from build123d import *

# Parameters (mm, degrees)
MODEL_R             = 1.25
BOSS_EXTRUDE1_DEPTH = 30
SKETCH1_R           = 2
BOSS_EXTRUDE3_DEPTH = 33
SKETCH3_W           = 38.889950408
SKETCH3_H           = 20
BOSS_EXTRUDE6_DEPTH = 3


with BuildPart() as part:
    # Model → Boss-Extrude1 (new body)
    with BuildSketch(Plane.XY):
        Polygon((29.652943866, 16.209286981), (29.652943866, 56.209286981), (19.652943866, 66.209286981), (16.11740996, 62.673753075), (24.652943866, 54.138219169), (24.652943866, 18.280354793), (16.11740996, 9.744820887), (19.652943866, 6.209286981), align=None)
        with Locations((22.885176913, 12.977053934)):
            Circle(MODEL_R, mode=Mode.SUBTRACT)
        with Locations((27.152943866, 36.209286981)):
            Circle(MODEL_R, mode=Mode.SUBTRACT)
        with Locations((22.885176913, 59.441520028)):
            Circle(MODEL_R, mode=Mode.SUBTRACT)
    extrude(amount=BOSS_EXTRUDE1_DEPTH)

    # Sketch1 → Boss-Extrude3 (add)
    with BuildSketch(Plane(origin=(0, 0, 0), x_dir=(-1, 0, 0), z_dir=(0, 0, -1))):
        Polygon((-37.652943866, 28.709286981), (-76.542894274, 28.709286981), (-76.542894274, 48.709286981), (-84.542894274, 48.709286981), (-84.542894274, 23.709286981), (-76.542894274, 23.709286981), (-29.652943866, 23.709286981), (-29.652943866, 28.709286981), (-29.652943866, 48.709286981), (-37.652943866, 48.709286981), align=None)
        with Locations((-80.542894274, 33.709286981)):
            Circle(SKETCH1_R, mode=Mode.SUBTRACT)
        with Locations((-80.542894274, 43.709286981)):
            Circle(SKETCH1_R, mode=Mode.SUBTRACT)
        with Locations(Location((-33.652943866, 33.709286981, 0), (0, 0, 180))):
            Circle(SKETCH1_R, mode=Mode.SUBTRACT)
        with Locations(Location((-33.652943866, 43.709286981, 0), (0, 0, 180))):
            Circle(SKETCH1_R, mode=Mode.SUBTRACT)
    extrude(amount=-BOSS_EXTRUDE3_DEPTH)

    # Sketch3 → Boss-Extrude6 (add)
    with BuildSketch(Plane.XY.offset(33)):
        with Locations((57.09791907, 38.709286981)):
            Rectangle(SKETCH3_W, SKETCH3_H)
    extrude(amount=-BOSS_EXTRUDE6_DEPTH)


solid = part.part
Can you work these out from the model? Positions are in its coordinate system, mm. A direction names the side the tool comes from. Give positions to 0.01 mm unless a question says otherwise; leave off trailing zeros. Loops run counter-clockwise (first coordinate to the right, second up) from the corner with the lowest first, then second, coordinate; pieces in that order, holes last. Notation, with made-up numbers: (-25, 58.5) -> (6, 58.5) arc R15 cw to (6, 85.5) -> close; hole circle Ø9 at (73, 48). An arc over 180 degrees is marked (long way). Use one line per item in the form item = value.
1) Will these pins go through, and if not, where does the flat tip stop? pin 1 (3 mm diameter, centred on x = 22.89, y = 59.44, fed in from -Z); pin 2 (3 mm diameter, centred on x = 37.5, z = 11.5, fed in from +Y); pin 3 (2 mm diameter, centred on y = 21.5, z = 9, fed in from +X); pin 4 (10 mm diameter, centred on x = 57.5, y = 42.5, fed in from -Z).
Answers:
pin_1 = 0
pin_2 = 48.71
pin_3 = 29.65
pin_4 = 30
2) If we section it at B-B (x = 33): Please give me the cut outline in (y, z), plus the area to 3 significant figures.
Answers:
outline = (23.71, 0) -> (31.82, 0) -> (31.82, 33) -> (23.71, 33) -> close; (35.6, 0) -> (41.82, 0) -> (41.82, 33) -> (35.6, 33) -> close; (45.6, 0) -> (48.71, 0) -> (48.71, 33) -> (45.6, 33) -> close
area = 575 mm²
3) We'd pull the mould along X, two halves only. Please class faces 1 (the face through (24.583, 11.139, 14.79)), 2 (the face through (76.543, 39, 15)), 3 (the face through (25.8, 36.6, 30)): released by +X, released by -X, zero draft, split by the parting line, or undercut.
Answers:
face_1 = released by +X
face_2 = undercut
face_3 = zero draft
4) If we section it at C-C (x = 61.5): Please give me the cut outline in (y, z).
Answers:
outline = (23.71, 0) -> (28.71, 0) -> (28.71, 30) -> (48.71, 30) -> (48.71, 33) -> (23.71, 33) -> close
5) I need wall thicknesses on line 1 along Y through (x, z) = (80.5, 22); line 2 along X through (y, z) = (39, 28); line 3 along Y through (x, z) = (30, 5.5). Which ranges of each line are inside material? Lowest first, please.
Answers:
line_1 = 23.71 to 31.71, 35.71 to 41.71, 45.71 to 48.71
line_2 = 24.65 to 37.65, 76.54 to 84.54
line_3 = 23.71 to 48.71
6) If we section it at A-A (z = 31.5): Please give me the cut outline in (x, y), plus the area to 3 significant figures.
Answers:
outline = (29.65, 23.71) -> (84.54, 23.71) -> (84.54, 48.71) -> (29.65, 48.71) -> close; hole circle Ø4 at (33.65, 33.71); hole circle Ø4 at (33.65, 43.71); hole circle Ø4 at (80.54, 33.71); hole circle Ø4 at (80.54, 43.71)
area = 1,320 mm²
7) For faces 4 (the face through (20.44, 14.07, 14.79)), 5 (the face through (57, 28.709, 15)), 6 (the face through (57, 48.709, 32)), 7 (the face through (29.653, 20, 15)), which set-ups out of +Z, -Z, +X, -X, +Y, -Y let a thin tool reach every point of the face, with its end or its side?
Answers:
face_4 = +Z, -Z, -X
face_5 = -Z, +Y
face_6 = +Z, -Z, +X, +Y
face_7 = +Z, -Z, +X, -Y
8) If we section it at D-D (y = 27.5): Please give me the cut outline in (x, z).
Answers:
outline = (24.65, 0) -> (84.54, 0) -> (84.54, 33) -> (29.65, 33) -> (29.65, 30) -> (24.65, 30) -> close
